Build history of the part. All positions in model axes, mm. A direction names the side the tool comes from. Give positions to 0.01 mm unless a question says otherwise; leave off trailing zeros. Write each loop counter-clockwise with the first axis right and the second up, starting at its lowest first coordinate (ties: lowest second). Pieces come first, ordered by that corner, then holes. Notation, with made-up numbers: (67.25, -38) -> (91.25, -38) arc R13 ccw to (91.25, -21) -> close; hole circle Ø7 at (-33.5, -26.5). An arc over 180 degrees is marked (long way). One line per question, with ' | ' between items. Start each with the question number.
(1) Band-saw the part on C-C, the plane x = 0.5. Give the cut face in (y, z), and give its area (3 significant figures).
(2) Drill centre lines: probe 1 along Y at (x, z) = (-17.5, 1.15); probe 2 along Y at (x, z) = (-7, 2.9); probe 3 along Z at (x, y) = (14.5, 2). Where is each one in solid material? Low to high. Write a range as from..to.
(3) Band-saw the part on B-B, the plane z = 0.55. Give the cut face in (x, y).
(4) Pin check, flat tips, straight feed: P1, Ø5, axis at x = 14, y = 5, coming from the -Z side; P2, Ø4, axis at x = -17.5, y = -7, coming from the +Z side; P3, Ø1.8, axis at y = 8.5, z = 2.5, coming from the -X side; P4, Ø1.5, axis at x = -15, z = 2.5, coming from the -Y side. Stop position of each tip, or through.
(5) Band-saw the part on A-A, the plane z = 2.8. Give the cut face in (x, y).
(6) Band-saw the part on D-D, the plane y = -1. Give the cut face in (x, z).
(7) Pull direction X, two halves, no side cores. Call faces 6 (the cylindrical face through (-19, -7, 1)), 7 (the flat face through (-15, 10.5, 1)), 8 (the flat face through (21, 0, 1)), 9 (the cylindrical face through (-19, 7, 1)): released by +X, released by -X, zero draft, split by the parting line, or undercut.
(8) Tool access for faces 1 (the flat face through (0, 4.303, 3)), 2 (the flat face through (-12.25, 7, 3)), 3 (the flat face through (12.25, 7, 3)), 4 (the flat face through (-15, -10.5, 1)), 5 (the cylindrical face through (16, -7, 1)): list every direction of +Z, -Z, +X, -X, +Y, -Y with a clear straight run to the whole face (end or side of a thin tool).
from build123d import *

# Parameters (mm, degrees)
SKETCH_R     = 1.5
PAD_DEPTH    = 1.5
SKETCH001_W  = 24.5
SKETCH001_H  = 6.196515
PAD001_DEPTH = 3.6


with BuildPart() as part:
    # Sketch → Pad (new body)
    with BuildSketch(Plane.XY):
        with BuildLine():
            ThreePointArc((-17.5, 10.5), (-19.974874, 9.474874), (-21, 7))
            Line((-21, -7), (-21, 7))
            ThreePointArc((-21, -7), (-19.974874, -9.474874), (-17.5, -10.5))
            Line((17.5, -10.5), (-17.5, -10.5))
            ThreePointArc((17.5, -10.5), (19.974874, -9.474874), (21, -7))
            Line((21, 7), (21, -7))
            ThreePointArc((21, 7), (19.974874, 9.474874), (17.5, 10.5))
            Line((-17.5, 10.5), (17.5, 10.5))
        make_face()
        with Locations((-17.5, 7)):
            Circle(SKETCH_R, mode=Mode.SUBTRACT)
        with Locations((-17.5, -7)):
            Circle(SKETCH_R, mode=Mode.SUBTRACT)
        with Locations((17.5, 7)):
            Circle(SKETCH_R, mode=Mode.SUBTRACT)
        with Locations((17.5, -7)):
            Circle(SKETCH_R, mode=Mode.SUBTRACT)
    extrude(amount=PAD_DEPTH)

    # Sketch001 → Pad001 (join)
    with BuildSketch(Plane.XY):
        with Locations((0, 7.401743)):
            Rectangle(SKETCH001_W, SKETCH001_H)
        with Locations((0, -7.401743)):
            Rectangle(SKETCH001_W, SKETCH001_H)
    extrude(amount=PAD001_DEPTH)


solid = part.part
Results:
1) outline: (-10.5, 0) -> (10.5, 0) -> (10.5, 3.6) -> (4.3, 3.6) -> (4.3, 1.5) -> (-4.3, 1.5) -> (-4.3, 3.6) -> (-10.5, 3.6) -> close | area: 57.5 mm²
2) probe 1: y = -10.5..-8.5, -5.5..5.5, 8.5..10.5 | probe 2: y = -10.5..-4.3, 4.3..10.5 | probe 3: z = 0..1.5
3) outline: (-21, -7) arc R3.5 ccw to (-17.5, -10.5) -> (17.5, -10.5) arc R3.5 ccw to (21, -7) -> (21, 7) arc R3.5 ccw to (17.5, 10.5) -> (-17.5, 10.5) arc R3.5 ccw to (-21, 7) -> close; hole circle Ø3 at (-17.5, -7); hole circle Ø3 at (-17.5, 7); hole circle Ø3 at (17.5, -7); hole circle Ø3 at (17.5, 7)
4) P1: stops at z = 0 | P2: stops at z = 1.5 | P3: stops at x = -12.25 | P4: passes through
5) outline: (-12.25, -10.5) -> (12.25, -10.5) -> (12.25, -4.3) -> (-12.25, -4.3) -> close; (-12.25, 4.3) -> (12.25, 4.3) -> (12.25, 10.5) -> (-12.25, 10.5) -> close
6) outline: (-21, 0) -> (21, 0) -> (21, 1.5) -> (-21, 1.5) -> close
7) face 6: undercut | face 7: zero draft | face 8: released by +X | face 9: undercut
8) face 1: +Z, +X, -X | face 2: +Z, -X, +Y, -Y | face 3: +Z, +X, +Y, -Y | face 4: +Z, -Z, +X, -X, -Y | face 5: +Z, -Z
